```python
from build123d import *

# Parameters (mm, degrees)
WHEEL_EDGES_FILLET_R     = 3.81
SKETCH2_R                = 2.0066
F_4_MOUNTING_HOLES_DEPTH = 12.7


with BuildPart() as part:
    # Wheel Cross Section → Main Wheel Rev (revolve)
    with BuildSketch(Plane.XY):
        Polygon((0, 6.35), (0, -6.35), (-38.1, -6.35), (-38.1, -19.05), (-76.2, -19.05), (-76.2, 19.05), (-38.1, 19.05), (-38.1, 6.35), align=None)
    revolve(axis=Axis((0, 6.35, 0), (0, -1, 0)))

    # Wheel Edges Fillet
    wheel_edges_fillet_edges = [part.edges().sort_by_distance(p)[0] for p in [
        (38.1, 19.05, 0),
        (38.1, -19.05, 0),
        (76.2, -19.05, 0),
        (76.2, 19.05, 0),
    ]]
    fillet(wheel_edges_fillet_edges, radius=WHEEL_EDGES_FILLET_R)

    # Sketch2 → 4 Mounting Holes (cut)
    with BuildSketch(Plane(origin=(0, 6.35, 0), x_dir=(1, 0, 0), z_dir=(0, 1, 0))):
        with Locations(Location((-6.858, 6.858, 0), (0, 0, 180))):
            Circle(SKETCH2_R)
        with Locations(Location((6.858, 6.858, 0), (0, 0, 180))):
            Circle(SKETCH2_R)
        with Locations(Location((6.858, -6.858, 0), (0, 0, 180))):
            Circle(SKETCH2_R)
        with Locations(Location((-6.858, -6.858, 0), (0, 0, 180))):
            Circle(SKETCH2_R)
    extrude(amount=-F_4_MOUNTING_HOLES_DEPTH, mode=Mode.SUBTRACT)


solid = part.part
```
The model under review builds one solid part; all positions refer to its coordinate system, in mm. A direction names the side the tool comes from. Coordinates: 2 decimals unless noted, no trailing zeros. Order: outer loops, then holes, each group sorted by start corner. A loop starts at its lowest first (then second) coordinate and runs counter-clockwise, first axis right, second up. Notation, with made-up numbers: (-16, -30) -> (3, -30) arc R37 ccw to (3, 7) -> close; hole circle Ø3 at (-36, 32). An arc over 180 degrees is marked (long way). Answer in a Markdown table with one row per item. Add a question column.
Item 1: We need section A-A on z = 0. Write out the cut boundary in (x, y).
Item 2: Machinability: for faces 1 (the cylindrical face through (8.863, 0.089, 6.946)), 2 (the cylindrical face through (30.235, -10.857, 23.183)), 3 (the flat face through (1, 6.35, -1)), which of the approach directions +Z, -Z, +X, -X, +Y, -Y give a long, thin tool a straight path to every point of the face, cutting with its end or side? Answer none if there is none.
Item 3: To check wall thickness, follow probe 1 along X at (y, z) = (6, 8); probe 2 along Y at (x, z) = (-22, -1); probe 3 along X at (y, z) = (-9.75, 0). State the ranges of each line that lie inside material, in increasing order.
Item 4: We need section C-C on y = 11. Write out the cut boundary in (x, z).
Item 5: Clearance check with flat-ended pins moving along their axes: pin 1 (1.5 mm diameter, centred on x = -0.5, y = 11.5, fed in from +Z); pin 2 (23 mm diameter, centred on x = 16, z = 15.5, fed in from +Y); pin 3 (2.5 mm diameter, centred on x = -6.858, z = 6.858, fed in from +Y); pin 4 (5 mm diameter, centred on x = 6.858, z = -6.858, fed in from -Y). State where each tip first meets the part, or that it passes through.
Item 6: We need section B-B on x = 0. Write out the cut boundary in (y, z).
Item 7: Mouldability with a two-part tool opening along Z and no side actions: class faces 4 (the flat face through (-31, 19.05, 31)), 5 (the cylindrical face through (60.47, 0.213, 46.367)), 6 (the cylindrical face through (-4.853, 0.089, 6.946)), 7 (the cylindrical face through (8.863, 0.089, -6.77)) as +Z half, -Z half, draft (parallel to the pull), parting line (faces both ways), or undercut.
Final values:
| question | item | result |
|---|---|---|
| 1 | outline | (-76.2, -15.24) arc R3.81 ccw to (-72.39, -19.05) -> (-41.91, -19.05) arc R3.81 ccw to (-38.1, -15.24) -> (-38.1, -6.35) -> (38.1, -6.35) -> (38.1, -15.24) arc R3.81 ccw to (41.91, -19.05) -> (72.39, -19.05) arc R3.81 ccw to (76.2, -15.24) -> (76.2, 15.24) arc R3.81 ccw to (72.39, 19.05) -> (41.91, 19.05) arc R3.81 ccw to (38.1, 15.24) -> (38.1, 6.35) -> (-38.1, 6.35) -> (-38.1, 15.24) arc R3.81 ccw to (-41.91, 19.05) -> (-72.39, 19.05) arc R3.81 ccw to (-76.2, 15.24) -> close |
| 2 | face 1 | +Y, -Y |
| 2 | face 2 | -Y |
| 2 | face 3 | +Y |
| 3 | probe 1 | x = -75.78 to -8.51, -5.21 to 5.21, 8.51 to 75.78 |
| 3 | probe 2 | y = -6.35 to 6.35 |
| 3 | probe 3 | x = -76.2 to -38.1, 38.1 to 76.2 |
| 4 | outline | circle Ø152.4 at (0, 0); hole circle Ø76.2 at (0, 0) |
| 5 | pin 1 | stops at z = 76.2 |
| 5 | pin 2 | stops at y = 6.35 |
| 5 | pin 3 | passes through |
| 5 | pin 4 | stops at y = -6.35 |
| 6 | outline | (-19.05, -72.39) arc R3.81 ccw to (-15.24, -76.2) -> (15.24, -76.2) arc R3.81 ccw to (19.05, -72.39) -> (19.05, -41.91) arc R3.81 ccw to (15.24, -38.1) -> (6.35, -38.1) -> (6.35, 38.1) -> (15.24, 38.1) arc R3.81 ccw to (19.05, 41.91) -> (19.05, 72.39) arc R3.81 ccw to (15.24, 76.2) -> (-15.24, 76.2) arc R3.81 ccw to (-19.05, 72.39) -> (-19.05, 41.91) arc R3.81 ccw to (-15.24, 38.1) -> (-6.35, 38.1) -> (-6.35, -38.1) -> (-15.24, -38.1) arc R3.81 ccw to (-19.05, -41.91) -> close |
| 7 | face 4 | draft |
| 7 | face 5 | parting line |
| 7 | face 6 | undercut |
| 7 | face 7 | undercut |
